Can you work these out from the drawing? Everything is in mm from the part's minimum corner. A direction names the side the tool comes from. Give positions to 0.01 mm unless a question says otherwise; leave off trailing zeros. Write each loop counter-clockwise with the first axis right and the second up, starting at its lowest first coordinate (ties: lowest second). Pieces come first, ordered by that corner, then holes. Notation, with made-up numbers: (49, -34) - (55, -34) arc R29 ccw to (55, -1) - close; hole circle Ø9 at (71, 70.25). An arc over 180 degrees is marked (long way). Return JSON: item names as keys, results as strings. Group by question number.
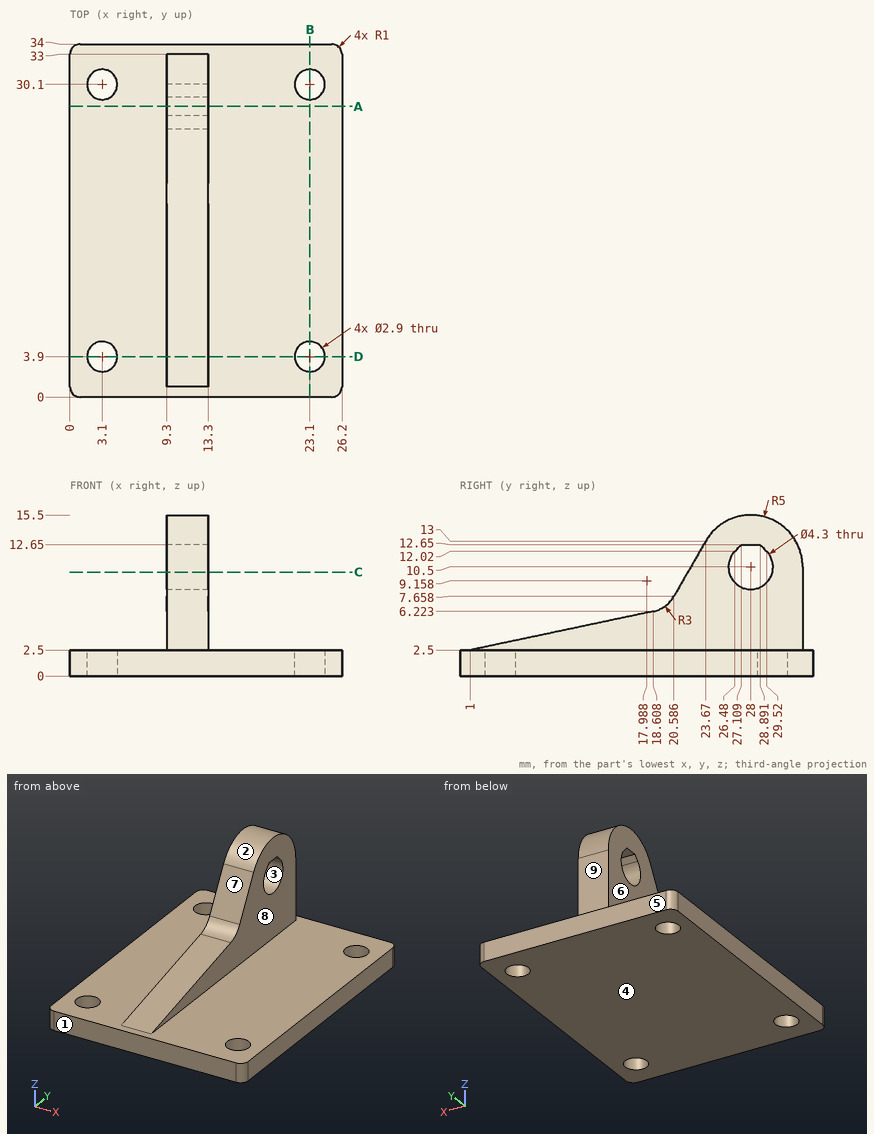
1) On a 3-axis mill with a long thin cutter (end or side, diameter ignored), from which of +Z, -Z, +X, -X, +Y, -Y can I reach the whole of each face in a straight line? I mean the marked faces 5, 6, 7, 8 and 9. Say none if no direction works.
2) Imagine slicing it at A-A, the plane y = 28. Write out the boundary of the cut face in (x, z).
3) We'd pull the mould along Z, two halves only. Please class the marked faces 1, 2, 3 and 4: pulls with the +Z half, pulls with the -Z half, needs draft (parallel to the pull), parting line crosses it, or undercut.
4) Will these pins go through, and if not, where does the flat tip stop? pin 1 Ø4 at (y, z) = (23.5, 7) entering from +X; pin 2 Ø3 at (x, z) = (12, 8) entering from +Y; pin 3 Ø4 at (x, y) = (3.1, 30.1) entering from +Z.
5) Imagine slicing it at B-B, the plane x = 23.1. Write out the boundary of the cut face in (y, z).
6) Imagine slicing it at C-C, the plane z = 10. Write out the boundary of the cut face in (x, y).
7) Imagine slicing it at D-D, the plane y = 3.9. Write out the boundary of the cut face in (x, z).
8) I need wall thicknesses on line 1 along Y through (x, z) = (3.1, 0.6); line 2 along Z through (x, y) = (22.5, 22.5); line 3 along X through (y, z) = (27, 7). Which ranges of each line are inside material? Lowest first, please.
Resolved:
{
 "1": {"face 5": "+Z, -Z, +X, -X, +Y", "face 6": "+Z, -X, +Y, -Y", "face 7": "+Z, +X, -X, -Y", "face 8": "+Z, +X, +Y, -Y", "face 9": "+Z, +X, -X, +Y"},
 "2": {"outline": "(0, 0) - (26.2, 0) - (26.2, 2.5) - (13.3, 2.5) - (13.3, 8.35) - (9.3, 8.35) - (9.3, 2.5) - (0, 2.5) - close; (9.3, 12.65) - (13.3, 12.65) - (13.3, 15.5) - (9.3, 15.5) - close"},
 "3": {"face 1": "needs draft", "face 2": "pulls with the +Z half", "face 3": "undercut", "face 4": "pulls with the -Z half"},
 "4": {"pin 1": "x = 13.3", "pin 2": "y = 33", "pin 3": "z = 2.5"},
 "5": {"outline": "(0, 0) - (2.45, 0) - (2.45, 2.5) - (0, 2.5) - close; (5.35, 0) - (28.65, 0) - (28.65, 2.5) - (5.35, 2.5) - close; (31.55, 0) - (34, 0) - (34, 2.5) - (31.55, 2.5) - close"},
 "6": {"outline": "(9.3, 21.94) - (13.3, 21.94) - (13.3, 25.91) - (9.3, 25.91) - close; (9.3, 30.09) - (13.3, 30.09) - (13.3, 33) - (9.3, 33) - close"},
 "7": {"outline": "(0, 0) - (1.65, 0) - (1.65, 2.5) - (0, 2.5) - close; (4.55, 0) - (21.65, 0) - (21.65, 2.5) - (13.3, 2.5) - (13.3, 3.11) - (9.3, 3.11) - (9.3, 2.5) - (4.55, 2.5) - close; (24.55, 0) - (26.2, 0) - (26.2, 2.5) - (24.55, 2.5) - close"},
 "8": {"line 1": "0 to 2.45, 5.35 to 28.65, 31.55 to 34", "line 2": "0 to 2.5", "line 3": "9.3 to 13.3"}
}
